CAD build for the part. Positions are in the model's coordinates, mm. Face numbers are marked on the shaded views. A direction names the side the tool comes from. Round coordinates to 2 decimals unless told otherwise and drop trailing zeros. Order: outer loops, then holes, each group sorted by start corner. A loop starts at its lowest first (then second) coordinate and runs counter-clockwise, first axis right, second up. Notation, with made-up numbers: (59.25, -1.75) - (117.25, -1.75) arc R24 ccw to (117.25, 25.25) - close; hole circle Ø2 at (-11.75, 86.25). An arc over 180 degrees is marked (long way). Write item = value, one per line.
from build123d import *

# Parameters (mm, degrees)
F0_R     = 12.7
F1_DEPTH = 16.51
F2_R     = 6.35
F3_DEPTH = 12.7
F4_R     = 6.35
F5_DEPTH = 12.7


with BuildPart() as f1:
    # F0 (on Front) → F1 (new body, symmetric)
    with BuildSketch(Plane.XZ):
        Circle(F0_R)
    extrude(amount=F1_DEPTH, both=True)

    # F2 (on face) → F3 (join)
    with BuildSketch(Plane.XZ.offset(16.51)):
        with BuildLine():
            Line((12.7, -1e-06), (12.699999, 38.099999))
            ThreePointArc((12.699999, 38.099999), (0, 50.8), (-12.700001, 38.1))
            Line((-12.700001, 38.1), (-12.7, 0))
            ThreePointArc((-12.7, 0), (0, -12.7), (12.7, -1e-06))
        make_face()
        Circle(F2_R, mode=Mode.SUBTRACT)
        with Locations((-1e-06, 38.1)):
            Circle(F2_R, mode=Mode.SUBTRACT)
    extrude(amount=F3_DEPTH)

    # F4 (on face) → F5 (join)
    with BuildSketch(Plane(origin=(0, 16.51, 0), x_dir=(-1, 0, 0), z_dir=(0, 1, 0))):
        with BuildLine():
            Line((12.7, -1e-06), (12.699999, 38.099999))
            ThreePointArc((12.699999, 38.099999), (0, 50.8), (-12.700001, 38.1))
            Line((-12.700001, 38.1), (-12.7, 0))
            ThreePointArc((-12.7, 0), (0, -12.7), (12.7, -1e-06))
        make_face()
        Circle(F4_R, mode=Mode.SUBTRACT)
        with Locations((-1e-06, 38.1)):
            Circle(F4_R, mode=Mode.SUBTRACT)
    extrude(amount=F5_DEPTH)


solid = f1.part
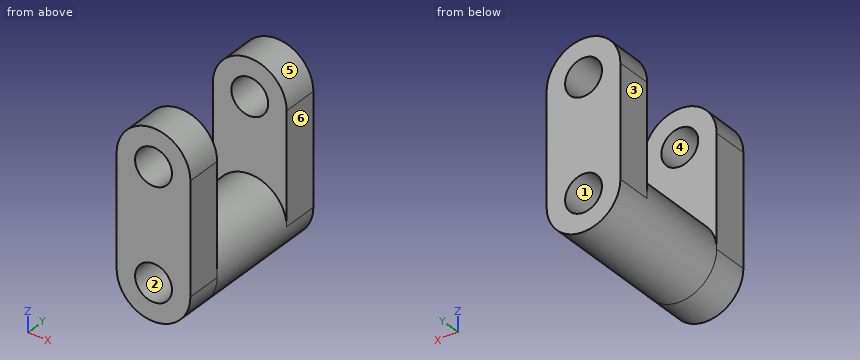
(1) Band-saw the part on D-D on z = -2. List the corners of the cut face in (x, y), plus the area to 3 significant figures.
Solved:
outline = (-12.54, -29.21) - (-6.03, -29.21) - (-6.03, -16.51) - (6.03, -16.51) - (6.03, -29.21) - (12.54, -29.21) - (12.54, 29.21) - (6.03, 29.21) - (6.03, 16.51) - (-6.03, 16.51) - (-6.03, 29.21) - (-12.54, 29.21) - close
area = 1,160 mm²
(2) Band-saw the part on A-A on z = 25.5. List the corners of the cut face in (x, y).
Solved:
outline = (-12.7, -29.21) - (12.7, -29.21) - (12.7, -16.51) - (-12.7, -16.51) - close; (-12.7, 16.51) - (12.7, 16.51) - (12.7, 29.21) - (-12.7, 29.21) - close
(3) Band-saw the part on B-B on x = 0. List the corners of the cut face in (y, z), plus the area to 3 significant figures.
Solved:
outline = (-29.21, -12.7) - (29.21, -12.7) - (29.21, -6.35) - (16.51, -6.35) - (16.51, 6.35) - (29.21, 6.35) - (29.21, 31.75) - (16.51, 31.75) - (16.51, 12.7) - (-16.51, 12.7) - (-16.51, 31.75) - (-29.21, 31.75) - (-29.21, 6.35) - (-16.51, 6.35) - (-16.51, -6.35) - (-29.21, -6.35) - close; (-29.21, 44.45) - (-16.51, 44.45) - (-16.51, 50.8) - (-29.21, 50.8) - close; (16.51, 44.45) - (29.21, 44.45) - (29.21, 50.8) - (16.51, 50.8) - close
area = 1,810 mm²
(4) Drop flat-ended pins along their axis: pin 1 (4 mm diameter, centred on x = -6.5, y = -2.5, fed in from -Z); pin 2 (11.5 mm diameter, centred on x = 0, z = 0, fed in from +Y); pin 3 (8 mm diameter, centred on x = -5, y = 8, fed in from +Z). Give the stop position or say it passes through.
Solved:
pin_1 = -11.88
pin_2 = 16.51
pin_3 = 12.66
(5) Pull direction Z, two halves, no side cores. Call the marked faces 4, 5 and 6: released by +Z, released by -Z, zero draft, split by the parting line, or undercut.
Solved:
face_4 = undercut
face_5 = released by +Z
face_6 = zero draft
(6) Tool access for the marked faces 1, 2 and 3: list every direction of +Z, -Z, +X, -X, +Y, -Y with a clear straight run to the whole face (end or side of a thin tool).
Solved:
face_1 = +Y
face_2 = -Y
face_3 = +Z, -Z, -X, +Y, -Y
(7) Probe line 1 along Z through (x, y) = (0, -26.25); line 2 along X through (y, z) = (-21, 38); line 3 along Z through (x, y) = (-5.25, 21.5). List the from-to ranges inside material, lowest first.
Solved:
line_1 = -12.7 to -6.35, 6.35 to 31.75, 44.45 to 50.8
line_2 = -12.7 to -6.35, 6.35 to 12.7
line_3 = -11.56 to -3.57, 3.57 to 34.53, 41.67 to 49.66
(8) Band-saw the part on C-C on y = -17.5. List the corners of the cut face in (x, z).
Solved:
outline = (-12.7, 0) arc R12.7 ccw to (12.7, 0) - (12.7, 38.1) arc R12.7 ccw to (-12.7, 38.1) - close; hole circle Ø12.7 at (0, 0); hole circle Ø12.7 at (0, 38.1)
